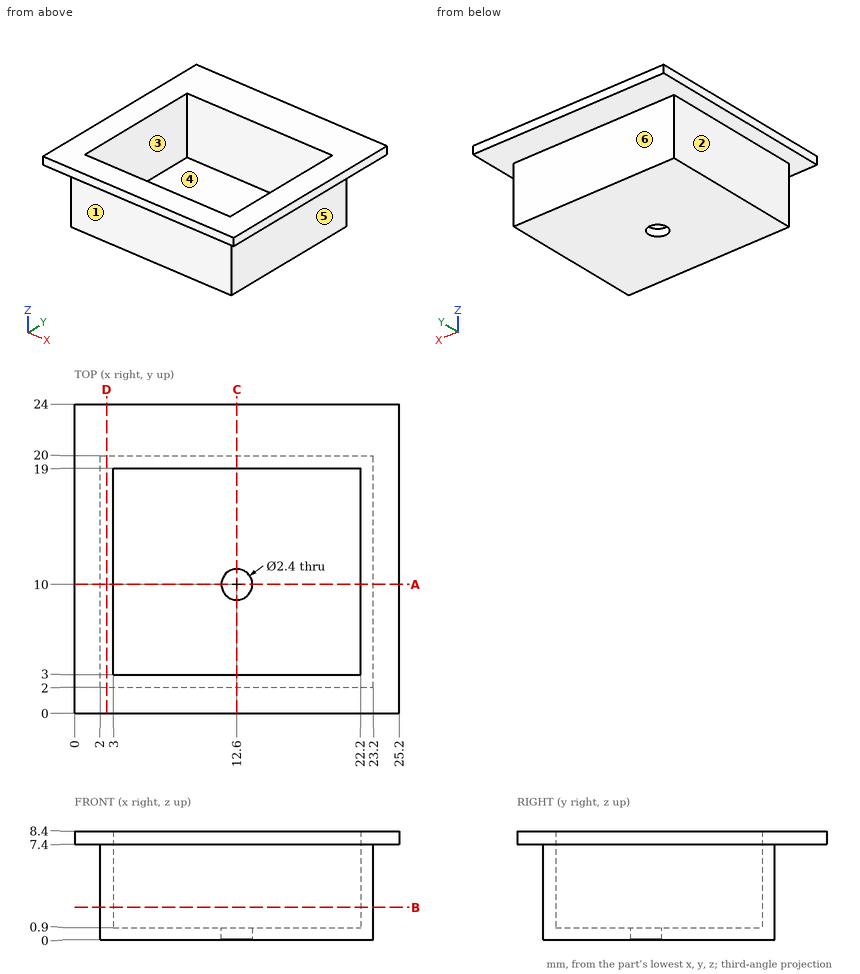
Verification items for this drawing (mm, ordinates from the low corner). A direction names the side the tool comes from. Round coordinates to 2 decimals unless told otherwise and drop trailing zeros. Loops run counter-clockwise (first coordinate to the right, second up) from the corner with the lowest first, then second, coordinate; pieces in that order, holes last. Notation, with made-up numbers: (81, -36.75) -> (88, -36.75) arc R22 cw to (88, -30.75) -> close; hole circle Ø3 at (14.5, 41). An arc over 180 degrees is marked (long way). Answer in a Markdown table with one row per item.
Q1. Thickness scan on L1, parallel to X at y = 13.25, z = 1.5; L2, parallel to Y at x = 12.6, z = 0.45; L3, parallel to Y at x = 13, z = 7.5. Record the ranges inside material, lowest first.
Data:
| item | result |
|---|---|
| L1 | x = 2 to 3, 22.2 to 23.2 |
| L2 | y = 2 to 8.8, 11.2 to 20 |
| L3 | y = 0 to 3, 19 to 24 |
Q2. Release check for a two-part mould opening along Y. For the marked faces 1, 2 and 3 record: released by +Y, released by -Y, zero draft, split by the parting line, or undercut.
Data:
| item | result |
|---|---|
| face 1 | released by -Y |
| face 2 | zero draft |
| face 3 | undercut |
Q3. Set-up check for the marked faces 4, 5 and 6: record each of +Z, -Z, +X, -X, +Y, -Y from which the full face is reachable in a straight line by a thin tool's end or side.
Data:
| item | result |
|---|---|
| face 4 | +Z |
| face 5 | -Z, +X, +Y, -Y |
| face 6 | -Z, +X, -X, +Y |
Q4. Go/stop test with flat-tipped pins: P1, Ø2, axis at y = 12.5, z = 2, coming from the -X side; P2, Ø1, axis at x = 6.5, z = 2.5, coming from the +Y side; P3, Ø4, axis at x = 10.5, z = 4, coming from the -Y side; P4, Ø2, axis at x = 12.6, y = 10, coming from the +Z side. Record where each tip stops, or that it passes through.
Data:
| item | result |
|---|---|
| P1 | stops at x = 2 |
| P2 | stops at y = 20 |
| P3 | stops at y = 2 |
| P4 | passes through |
Q5. Sectioned sample at A-A on y = 10. Enter the section's corners in (x, z).
Data:
| item | result |
|---|---|
| outline | (0, 7.4) -> (2, 7.4) -> (2, 0) -> (11.4, 0) -> (11.4, 0.9) -> (3, 0.9) -> (3, 8.4) -> (0, 8.4) -> close; (13.8, 0) -> (23.2, 0) -> (23.2, 7.4) -> (25.2, 7.4) -> (25.2, 8.4) -> (22.2, 8.4) -> (22.2, 0.9) -> (13.8, 0.9) -> close |
Q6. Sectioned sample at D-D on x = 2.5. Enter the section's corners in (y, z).
Data:
| item | result |
|---|---|
| outline | (0, 7.4) -> (2, 7.4) -> (2, 0) -> (20, 0) -> (20, 7.4) -> (24, 7.4) -> (24, 8.4) -> (0, 8.4) -> close |
Q7. Sectioned sample at B-B on z = 2.5. Enter the section's corners in (x, y), then the cut area to 3 significant figures.
Data:
| item | result |
|---|---|
| outline | (2, 2) -> (23.2, 2) -> (23.2, 20) -> (2, 20) -> close; hole (3, 3) -> (22.2, 3) -> (22.2, 19) -> (3, 19) -> close |
| area | 74.4 mm^2 |
Q8. Sectioned sample at C-C on x = 12.6. Enter the section's corners in (y, z).
Data:
| item | result |
|---|---|
| outline | (0, 7.4) -> (2, 7.4) -> (2, 0) -> (8.8, 0) -> (8.8, 0.9) -> (3, 0.9) -> (3, 8.4) -> (0, 8.4) -> close; (11.2, 0) -> (20, 0) -> (20, 7.4) -> (24, 7.4) -> (24, 8.4) -> (19, 8.4) -> (19, 0.9) -> (11.2, 0.9) -> close |
